from build123d import *

# Parameters (mm, degrees)
SKETCH2_R                 = 0.315
CUT_EXTRUDE1_DEPTH        = 4
SKETCH3_R                 = 0.425
CUT_EXTRUDE2_DEPTH        = 37.233654202
SKETCH4_R                 = 0.635
CUT_EXTRUDE3_DEPTH        = 37.16349315
FILLET1_R                 = 1.25
M2X0_4_TAPPED_HOLE1_D     = 1.6
M2X0_4_TAPPED_HOLE1_DEPTH = 6.35
M2X0_4_TAPPED_HOLE1_TIP   = 0.480688495


with BuildPart() as part:
    # Sketch1 → Revolve1 (revolve)
    with BuildSketch(Plane.XY):
        Polygon((0, 23.7871), (0, 7.5), (13.272, 7.5), (13.272, 11.25), (17.272, 11.25), (17.272, 18.7071), (3.81, 18.7071), (3.81, 23.7871), align=None)
    revolve(axis=Axis((13.272, 0, 0), (-1, 0, 0)))

    # Sketch2 → Cut-Extrude1 (cut)
    with BuildSketch(Plane(origin=(17.272, 0, 0), x_dir=(0, 0, -1), z_dir=(1, 0, 0))):
        with BuildLine():
            Line((-0.657808531, -0.677910665), (0, 0))
            Line((0, 0), (-0.494974747, 0.494974747))
            Line((-0.494974747, 0.494974747), (-8.434511887, -7.444562393))
            ThreePointArc((-8.434511887, -7.444562393), (-7.954951288, -7.954951288), (-7.444562393, -8.434511887))
            Line((-7.444562393, -8.434511887), (-0.16558691, -1.155536403))
            Line((-0.16558691, -1.155536403), (-0.657808531, -0.677910665))
        make_face()
        with BuildLine():
            Line((-12.723678558, -13.713628052), (-7.444562393, -8.434511887))
            ThreePointArc((-7.444562393, -8.434511887), (-7.954951288, -7.954951288), (-8.434511887, -7.444562393))
            Line((-8.434511887, -7.444562393), (-13.713628052, -12.723678558))
            ThreePointArc((-13.713628052, -12.723678558), (-13.473131789, -12.978070358), (-13.227917265, -13.227917267))
            ThreePointArc((-13.227917265, -13.227917267), (-12.978070357, -13.473131789), (-12.723678558, -13.713628052))
        make_face()
        with BuildLine():
            Line((13.738626304, -12.696682153), (8.384270986, -7.501099921))
            ThreePointArc((8.384270986, -7.501099921), (7.901171337, -8.00837009), (7.387437256, -8.484590196))
            Line((7.387437256, -8.484590196), (12.750537979, -13.688658505))
            ThreePointArc((12.750537979, -13.688658505), (13.09218126, -13.362274517), (13.425472665, -13.027366354))
            ThreePointArc((13.425472665, -13.027366354), (13.58305585, -12.862977268), (13.738626304, -12.696682153))
        make_face()
        with BuildLine():
            Line((8.384270986, -7.501099921), (0.317132147, 0.326823466))
            Line((0.317132147, 0.326823466), (0, 0))
            Line((0, 0), (0.494974747, -0.494974747))
            Line((0.494974747, -0.494974747), (-0.16558691, -1.155536403))
            Line((-0.16558691, -1.155536403), (7.387437256, -8.484590196))
            ThreePointArc((7.387437256, -8.484590196), (7.901171337, -8.00837009), (8.384270986, -7.501099921))
        make_face()
        with Locations((0, -14.9775)):
            Circle(SKETCH2_R)
        with Locations((-12.970895485, 7.48875)):
            Circle(SKETCH2_R)
        with Locations((12.970895485, 7.48875)):
            Circle(SKETCH2_R)
    extrude(amount=-CUT_EXTRUDE1_DEPTH, mode=Mode.SUBTRACT)

    # Sketch3 → Cut-Extrude2 (cut, through all)
    with BuildSketch(Plane(origin=(3.81, 0, 0), x_dir=(0, 0, -1), z_dir=(1, 0, 0))):
        with Locations(Location((0, 21.082, 0), (0, 0, 90))):
            Circle(SKETCH3_R)
    extrude(amount=-CUT_EXTRUDE2_DEPTH, mode=Mode.SUBTRACT)

    # Sketch4 → Cut-Extrude3 (cut, through all)
    with BuildSketch(Plane(origin=(13.272, 0, 0), x_dir=(0, 0, -1), z_dir=(1, 0, 0))):
        with Locations(Location((0, 9.375, 0), (0, 0, 90))):
            Circle(SKETCH4_R)
        with Locations(Location((0, -9.375, 0), (0, 0, 90))):
            Circle(SKETCH4_R)
    extrude(amount=-CUT_EXTRUDE3_DEPTH, mode=Mode.SUBTRACT)

    # Fillet1
    fillet1_edges = [part.edges().sort_by_distance(p)[0] for p in [
        (15.272, -7.444562393, 8.434511887),
        (15.272, -8.434511887, 7.444562393),
        (15.272, -7.501099921, -8.384270986),
        (15.272, -8.484590196, -7.387437256),
    ]]
    fillet(fillet1_edges, radius=FILLET1_R)

    # M2x0.4 Tapped Hole1
    with Locations(Plane(origin=(17.272, 7.48875, 12.970895485), x_dir=(0, 0, 1), z_dir=(1, 0, 0))):
        with Locations((0, 0), (-25.94179097, 0), (-12.970895485, 22.46625)):
            Hole(M2X0_4_TAPPED_HOLE1_D / 2, depth=M2X0_4_TAPPED_HOLE1_DEPTH)
            with Locations((0, 0, -(M2X0_4_TAPPED_HOLE1_DEPTH + M2X0_4_TAPPED_HOLE1_TIP / 2))):  # 118° drill point
                Cone(0, M2X0_4_TAPPED_HOLE1_D / 2, M2X0_4_TAPPED_HOLE1_TIP, mode=Mode.SUBTRACT)


solid = part.part
Design review of the part built by this model. Coordinates are the model's own, in mm. A direction names the side the tool comes from. Round coordinates to 2 decimals unless told otherwise and drop trailing zeros. Write each loop counter-clockwise with the first axis right and the second up, starting at its lowest first coordinate (ties: lowest second). Pieces come first, ordered by that corner, then holes. Notation, with made-up numbers: (-28.75, 14) - (9.25, 14) arc R18 ccw to (9.25, 18) - close; hole circle Ø2 at (47.5, 53). An arc over 180 degrees is marked (long way). Use a Markdown table: item, result. Add a question column.
1. Wall thickness on probe 1 along Z at (x, y) = (14.3, 0); probe 2 along Z at (x, y) = (12.5, -5); probe 3 along X at (y, z) = (13, 19.5): over which ranges is each line inside the solid? List them lowest first.
2. We need section C-C (x = 12.5). State the section outline as (y, z) points (1 decimal).
3. We need section D-D (y = -16.5). State the section outline as (x, z) points.
4. Clearance check with flat-ended pins moving along their axes: pin 1 (6 mm diameter, centred on x = 7, y = -19, fed in from -Z); pin 2 (1 mm diameter, centred on y = -16.5, z = -15, fed in from +X); pin 3 (1.3 mm diameter, centred on y = 7.49, z = -12.97, fed in from +X); pin 4 (13.5 mm diameter, centred on y = 0, z = 0, fed in from +X). State where each tip first meets the part, or that it passes through.
5. For faces 1 (the face through (15.3, -10.45, 11.44)), 2 (the face through (17.272, 14, 0)), list the 3-axis set-ups (+Z, -Z, +X, -X, +Y, -Y) from which the entire face can be reached by the end or side of a thin tool; tool diameter is ignored.
6. We need section A-A (y = 0). State the section outline as (x, z) points.
7. We need section B-B (z = -1.5). State the section outline as (x, y) points, then the cut area to 3 significant figures.
Output:
| question | item | result |
|---|---|---|
| 1 | probe 1 | z = -18.71 to -11.25, 11.25 to 18.71 |
| 1 | probe 2 | z = -18.03 to -5.59, 5.59 to 18.03 |
| 1 | probe 3 | x = 0 to 3.81 |
| 2 | outline | circle Ø37.4 at (0, 0); hole circle Ø1.6 at (-15, 0); hole circle Ø1.3 at (-9.4, 0); hole circle Ø15 at (0, 0); hole circle Ø1.6 at (7.5, -13); hole circle Ø1.6 at (7.5, 13); hole circle Ø1.3 at (9.4, 0) |
| 3 | outline | (0, -17.13) - (3.81, -17.13) - (3.81, -8.82) - (17.27, -8.82) - (17.27, 8.82) - (3.81, 8.82) - (3.81, 17.13) - (0, 17.13) - close |
| 4 | pin 1 | stops at z = -9.69 |
| 4 | pin 2 | stops at x = 3.81 |
| 4 | pin 3 | stops at x = 10.83 |
| 4 | pin 4 | passes through |
| 5 | face 1 | +X |
| 5 | face 2 | +Z, -Z, +X, +Y, -Y |
| 6 | outline | (0, -23.79) - (3.81, -23.79) - (3.81, -18.71) - (17.27, -18.71) - (17.27, -11.25) - (13.27, -11.25) - (13.27, -7.5) - (0, -7.5) - close; (0, 7.5) - (13.27, 7.5) - (13.27, 11.25) - (17.27, 11.25) - (17.27, 18.71) - (3.81, 18.71) - (3.81, 23.79) - (0, 23.79) - close |
| 7 | outline | (0, -23.74) - (3.81, -23.74) - (3.81, -18.65) - (17.27, -18.65) - (17.27, -11.15) - (13.27, -11.15) - (13.27, -7.35) - (0, -7.35) - close; (0, 7.35) - (13.27, 7.35) - (13.27, 11.15) - (17.27, 11.15) - (17.27, 18.65) - (3.81, 18.65) - (3.81, 23.74) - (0, 23.74) - close |
| 7 | area | 399 mm2 |
